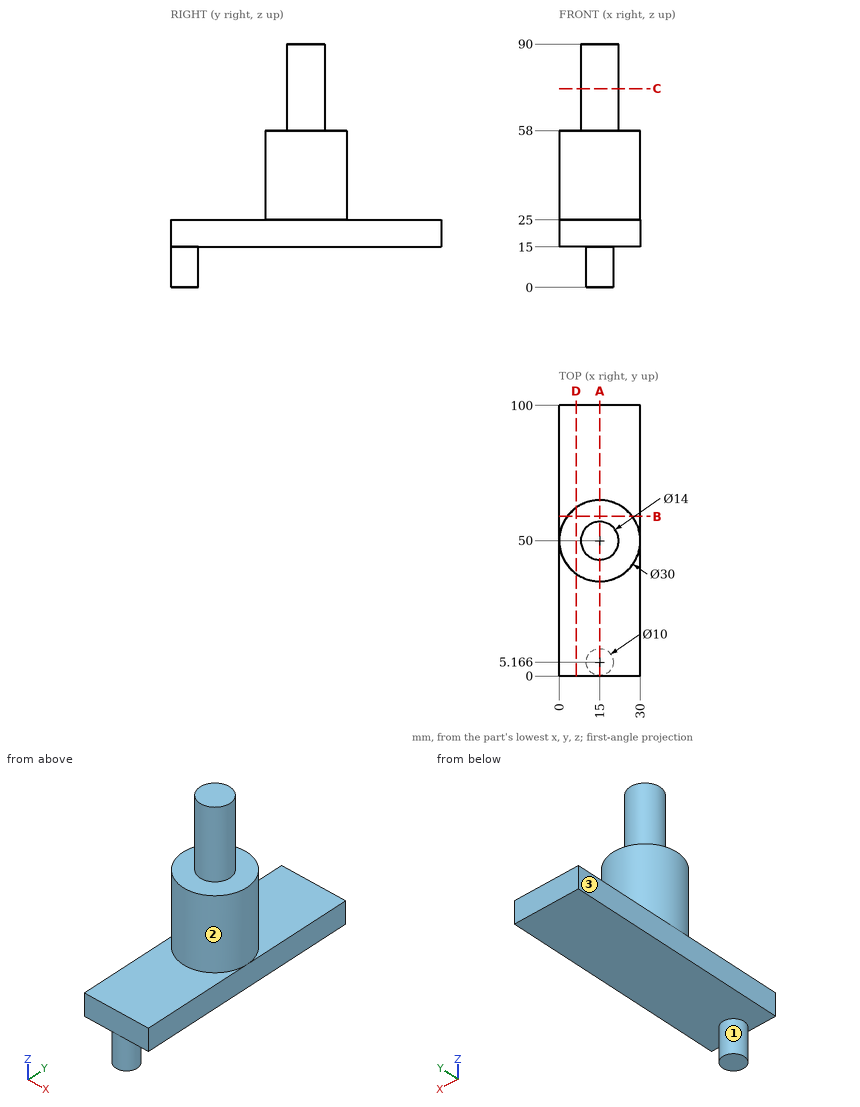
Geometry check sheet. Reference: drawing and pictorial views, mm from the part's lowest x, y, z. A direction names the side the tool comes from. Coordinates: 2 decimals unless noted, no trailing zeros. Loops run counter-clockwise (first coordinate to the right, second up) from the corner with the lowest first, then second, coordinate; pieces in that order, holes last. Notation, with made-up numbers: (27.5, -39.75) - (61.5, -39.75) arc R8 ccw to (61.5, -33.75) - close; hole circle Ø5 at (48, -23.5). An arc over 180 degrees is marked (long way). Return JSON: item names as keys, results as strings.
1. Thickness scan on L1, parallel to Z at x = 12.5, y = 32.5; L2, parallel to Z at x = 18.75, y = 6; L3, parallel to Y at x = 22.75, z = 55. Record the ranges inside material, lowest first.
Established:
{"L1": "z = 15 to 25", "L2": "z = 0 to 25", "L3": "y = 37.16 to 62.84"}
2. Section check C-C, the plane z = 73.5. Record the boundary of the cut face in (x, y), then the cut area to 3 significant figures.
Established:
{"outline": "circle Ø14 at (15, 50)", "area": "154 mm2"}
3. Tool access check on the marked faces 1, 2 and 3. Record the directions out of +Z, -Z, +X, -X, +Y, -Y that give a thin tool (end or side, any length) a straight path to the whole face; none if there is none.
Established:
{"face 1": "-Z", "face 2": "+Z", "face 3": "+Z, -Z, -X, +Y, -Y"}
4. Section check D-D, the plane x = 6.25. Record the boundary of the cut face in (y, z), then the cut area to 3 significant figures.
Established:
{"outline": "(0, 15) - (100, 15) - (100, 25) - (62.18, 25) - (62.18, 58) - (37.82, 58) - (37.82, 25) - (0, 25) - close", "area": "1,800 mm2"}
5. Section check A-A, the plane x = 15. Record the boundary of the cut face in (y, z).
Established:
{"outline": "(0, 15) - (0.17, 15) - (0.17, 0) - (10.17, 0) - (10.17, 15) - (100, 15) - (100, 25) - (65, 25) - (65, 58) - (57, 58) - (57, 90) - (43, 90) - (43, 58) - (35, 58) - (35, 25) - (0, 25) - close"}
6. Go/stop test with flat-tipped pins: pin 1 (15 mm diameter, centred on x = 14.5, y = 61, fed in from -Z); pin 2 (9 mm diameter, centred on x = 11.5, y = 19, fed in from +Z); pin 3 (8 mm diameter, centred on x = 18, z = 51, fed in from +Y); pin 4 (12 mm diameter, centred on y = 28, z = 54, fed in from +X). Record where each tip stops, or that it passes through.
Established:
{"pin 1": "stops at z = 15", "pin 2": "stops at z = 25", "pin 3": "stops at y = 65", "pin 4": "passes through"}
7. Section check B-B, the plane y = 59. Record the boundary of the cut face in (x, z), then the cut area to 3 significant figures.
Established:
{"outline": "(0, 15) - (30, 15) - (30, 25) - (27, 25) - (27, 58) - (3, 58) - (3, 25) - (0, 25) - close", "area": "1,090 mm2"}
